Check sheet for the drawn part. Datum: minimum x, y, z corner. Units: mm. Coordinates: 2 decimals unless noted, no trailing zeros. Write each loop counter-clockwise with the first axis right and the second up, starting at its lowest first coordinate (ties: lowest second). Pieces come first, ordered by that corner, then holes. Notation, with made-up numbers: M -5.75,29 L -0.75,29 A20 cw -0.75,39 Z; hole C -32.75,-14.5 d11. An arc over 180 degrees is marked long. Answer in a Markdown table with one row per item.
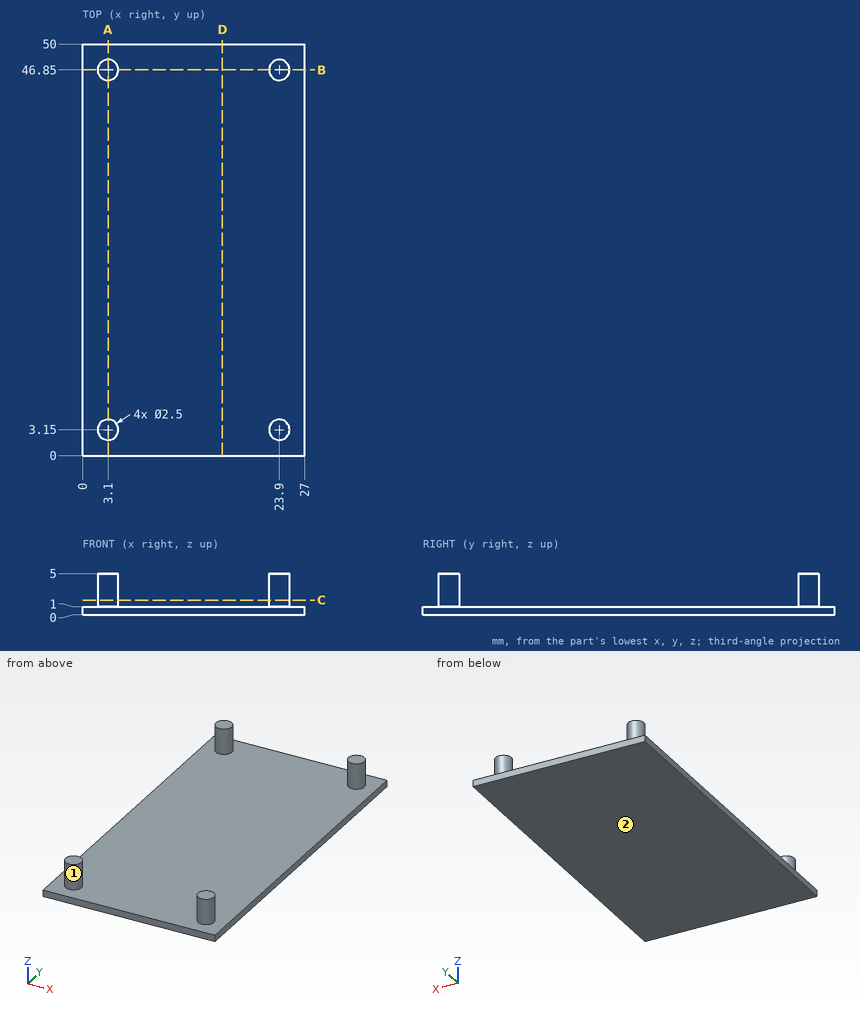
1) Sectioned sample at D-D (x = 17). Record the cut outline in (y, z).
Response values:
| item | result |
|---|---|
| outline | M 0,0 L 50,0 L 50,1 L 0,1 Z |
2) Thickness scan on L1, parallel to Y at x = 24, z = 1.85; L2, parallel to Z at x = 21, y = 48; L3, parallel to Y at x = 2.5, z = 3.4. Record the ranges inside material, lowest first. Write a range as [from, to].
Response values:
| item | result |
|---|---|
| L1 | y = [1.9, 4.4], [45.6, 48.1] |
| L2 | z = [0, 1] |
| L3 | y = [2.05, 4.25], [45.75, 47.95] |
3) Release check for a two-part mould opening along Y. For the marked faces 1 and 2 record: +Y half, -Y half, draft (parallel to the pull), parting line (faces both ways), or undercut.
Response values:
| item | result |
|---|---|
| face 1 | undercut |
| face 2 | draft |
4) Depth check by flat-ended pin: pin 1 (2 mm diameter, centred on x = 24, y = 25.5, fed in from +Z); pin 2 (1.5 mm diameter, centred on y = 42, z = 3, fed in from -X). Enter the tip coordinate at first touch or a pass-through.
Response values:
| item | result |
|---|---|
| pin 1 | stops at z = 1 |
| pin 2 | passes through |
5) Sectioned sample at B-B (y = 46.85). Record the cut outline in (x, z).
Response values:
| item | result |
|---|---|
| outline | M 0,0 L 27,0 L 27,1 L 25.15,1 L 25.15,5 L 22.65,5 L 22.65,1 L 4.35,1 L 4.35,5 L 1.85,5 L 1.85,1 L 0,1 Z |
6) Sectioned sample at A-A (x = 3.1). Record the cut outline in (y, z).
Response values:
| item | result |
|---|---|
| outline | M 0,0 L 50,0 L 50,1 L 48.1,1 L 48.1,5 L 45.6,5 L 45.6,1 L 4.4,1 L 4.4,5 L 1.9,5 L 1.9,1 L 0,1 Z |
7) Sectioned sample at C-C (z = 1.8). Record the cut outline in (x, y), then the cut area to 3 significant figures.
Response values:
| item | result |
|---|---|
| outline | C 3.1,3.15 d2.5; C 3.1,46.85 d2.5; C 23.9,3.15 d2.5; C 23.9,46.85 d2.5 |
| area | 19.6 mm² |
